from build123d import *

# Parameters (mm, degrees)
SKETCH1_R                       = 0.5
BOSS_EXTRUDE1_DEPTH             = 1.8
SKETCH2_R                       = 4
BOSS_EXTRUDE2_DEPTH             = 2.6
BOSS_EXTRUDE2_DIRECTION_2_REACH = 19.066
SKETCH3_R                       = 2
CUT_EXTRUDE1_DEPTH              = 18.531685601


with BuildPart() as part:
    # Sketch1 → Boss-Extrude1 (new body)
    with BuildSketch(Plane.XY):
        Polygon((-2.475, -12), (2.475, -12), (2.475, -2.475), (12, -2.475), (12, 2.475), (2.475, 2.475), (2.475, 12), (-2.475, 12), (-2.475, 2.475), (-12, 2.475), (-12, -2.475), (-2.475, -2.475), align=None)
        with Locations((0, 9.5)):
            Circle(SKETCH1_R, mode=Mode.SUBTRACT)
        with Locations((0, 7)):
            Circle(SKETCH1_R, mode=Mode.SUBTRACT)
        with Locations(Location((0, -9.5, 0), (0, 0, 180))):
            Circle(SKETCH1_R, mode=Mode.SUBTRACT)
        with Locations(Location((0, -7, 0), (0, 0, 180))):
            Circle(SKETCH1_R, mode=Mode.SUBTRACT)
        with Locations((-9.5, 0)):
            Circle(SKETCH1_R, mode=Mode.SUBTRACT)
        with Locations((-7, 0)):
            Circle(SKETCH1_R, mode=Mode.SUBTRACT)
        with Locations(Location((9.5, 0, 0), (0, 0, 180))):
            Circle(SKETCH1_R, mode=Mode.SUBTRACT)
        with Locations(Location((7, 0, 0), (0, 0, 180))):
            Circle(SKETCH1_R, mode=Mode.SUBTRACT)
    extrude(amount=BOSS_EXTRUDE1_DEPTH)

    # Sketch2 → Boss-Extrude2 (add)
    with BuildSketch(Plane.XY.offset(1.8)):
        Circle(SKETCH2_R)
    extrude(amount=BOSS_EXTRUDE2_DEPTH)

    # Boss-Extrude2 direction 2: up to this face of the body (flat: up to its plane)
    boss_extrude2_direction_2_end = Plane(part.part.faces().sort_by_distance((0, 0, 0))[0])
    # Sketch2 → Boss-Extrude2 direction 2 (add, up to the picked face)
    with BuildSketch(Plane.XY.offset(1.8), mode=Mode.PRIVATE) as boss_extrude2_direction_2_sk1:
        Circle(SKETCH2_R)
    boss_extrude2_direction_2_tool1 = split(extrude(boss_extrude2_direction_2_sk1.sketch, amount=-BOSS_EXTRUDE2_DIRECTION_2_REACH, mode=Mode.PRIVATE), bisect_by=boss_extrude2_direction_2_end, keep=Keep.BOTH, mode=Mode.PRIVATE)
    add(boss_extrude2_direction_2_tool1.solids().sort_by(Axis((0, 0, 1.8), (0, 0, -1)))[0])

    # Sketch3 → Cut-Extrude1 (cut, through all)
    with BuildSketch(Plane(origin=(0, 0, 0), x_dir=(-1, 0, 0), z_dir=(0, 0, -1))):
        Circle(SKETCH3_R)
    extrude(amount=-CUT_EXTRUDE1_DEPTH, mode=Mode.SUBTRACT)


solid = part.part
Design review of the part built by this model. Coordinates are the model's own, in mm. A direction names the side the tool comes from. Coordinates: 2 decimals unless noted, no trailing zeros. Write each loop counter-clockwise with the first axis right and the second up, starting at its lowest first coordinate (ties: lowest second). Pieces come first, ordered by that corner, then holes. Notation, with made-up numbers: (16, -29.75) - (62, -29.75) arc R27 ccw to (62, -6.75) - close; hole circle Ø8 at (-34.75, -15). An arc over 180 degrees is marked (long way). One line per item, written item: value.
1) To check wall thickness, follow probe 1 along Y at (x, z) = (0, 0.8); probe 2 along Y at (x, z) = (9.5, 0.65) (3 decimals); probe 3 along Y at (x, z) = (0, 2.85). State the ranges of each line that lie inside material, in increasing order.
Answer sheet:
probe 1: y = -12 to -10, -9 to -7.5, -6.5 to -2, 2 to 6.5, 7.5 to 9, 10 to 12
probe 2: y = -2.475 to -0.5, 0.5 to 2.475
probe 3: y = -4 to -2, 2 to 4
2) For faces 1 (the face through (-12, 0, 1)), 2 (the face through (-2.475, -8, 1)), 3 (the face through (-2, -1, 0)), 4 (the face through (-2.475, 8, 1)), 5 (the face through (2.475, 8, 1)), list the 3-axis set-ups (+Z, -Z, +X, -X, +Y, -Y) from which the entire face can be reached by the end or side of a thin tool; tool diameter is ignored.
Answer sheet:
face 1: +Z, -Z, -X, +Y, -Y
face 2: +Z, -Z, -X, -Y
face 3: -Z, +X, -X, +Y, -Y
face 4: +Z, -Z, -X, +Y
face 5: +Z, -Z, +X, +Y
3) Insertion check: pin 1 (0.5 mm diameter, centred on y = 8.5, z = 0.5, fed in from -X) (3 decimals); pin 2 (2 mm diameter, centred on y = 7.5, z = 2, fed in from +X) (3 decimals); pin 3 (0.5 mm diameter, centred on x = 6, z = 1, fed in from -Y) (3 decimals). Each pin has a flat end and moves straight along its axis. Give the tip position at first contact, or say it passes through.
Answer sheet:
pin 1: stops at x = -2.475
pin 2: stops at x = 2.475
pin 3: stops at y = -2.475
4) Add section B-B (y = 0). State the section outline as (x, z) points.
Answer sheet:
outline: (-12, 0) - (-10, 0) - (-10, 1.8) - (-12, 1.8) - close; (-9, 0) - (-7.5, 0) - (-7.5, 1.8) - (-9, 1.8) - close; (-6.5, 0) - (-2, 0) - (-2, 4.4) - (-4, 4.4) - (-4, 1.8) - (-6.5, 1.8) - close; (2, 0) - (6.5, 0) - (6.5, 1.8) - (4, 1.8) - (4, 4.4) - (2, 4.4) - close; (7.5, 0) - (9, 0) - (9, 1.8) - (7.5, 1.8) - close; (10, 0) - (12, 0) - (12, 1.8) - (10, 1.8) - close
5) Add section A-A (x = -9.5). State the section outline as (y, z) points (3 decimals).
Answer sheet:
outline: (-2.475, 0) - (-0.5, 0) - (-0.5, 1.8) - (-2.475, 1.8) - close; (0.5, 0) - (2.475, 0) - (2.475, 1.8) - (0.5, 1.8) - close
6) Mouldability with a two-part tool opening along Y and no side actions: class faces 6 (the face through (2.475, -8, 1)), 7 (the face through (-10, 0, 1)), 8 (the face through (0, -12, 1)) as +Y half, -Y half, draft (parallel to the pull), parting line (faces both ways), or undercut.
Answer sheet:
face 6: draft
face 7: undercut
face 8: -Y half
